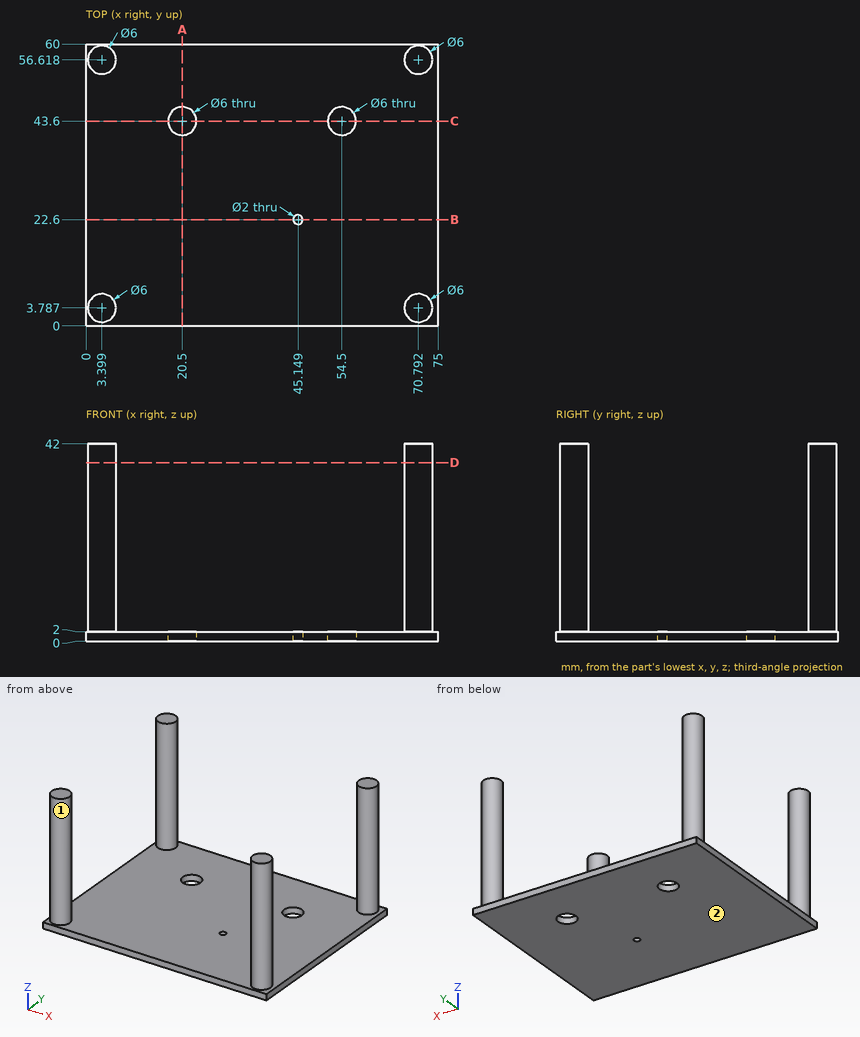
Verification items for this drawing (mm, ordinates from the low corner). Give positions to 0.01 mm unless a question says otherwise; leave off trailing zeros. Write each loop counter-clockwise with the first axis right and the second up, starting at its lowest first coordinate (ties: lowest second). Pieces come first, ordered by that corner, then holes. Notation, with made-up numbers: (-15, 79.5) -> (27, 79.5) arc R23 ccw to (27, 90.5) -> close; hole circle Ø4 at (44.25, 53). An arc over 180 degrees is marked (long way). Write item = value, one per line.
Item 1: Sectioned sample at A-A on x = 20.5. Record the boundary of the cut face in (y, z).
Output:
outline = (0, 0) -> (40.6, 0) -> (40.6, 2) -> (0, 2) -> close; (46.6, 0) -> (60, 0) -> (60, 2) -> (46.6, 2) -> close
Item 2: Sectioned sample at C-C on y = 43.6. Record the boundary of the cut face in (x, z).
Output:
outline = (0, 0) -> (17.5, 0) -> (17.5, 2) -> (0, 2) -> close; (23.5, 0) -> (51.5, 0) -> (51.5, 2) -> (23.5, 2) -> close; (57.5, 0) -> (75, 0) -> (75, 2) -> (57.5, 2) -> close
Item 3: Sectioned sample at D-D on z = 38. Record the boundary of the cut face in (x, y).
Output:
outline = circle Ø6 at (3.4, 3.79); circle Ø6 at (3.4, 56.62); circle Ø6 at (70.79, 3.79); circle Ø6 at (70.79, 56.62)
Item 4: Sectioned sample at B-B on y = 22.6. Record the boundary of the cut face in (x, z), and give its area (3 significant figures).
Output:
outline = (0, 0) -> (44.15, 0) -> (44.15, 2) -> (0, 2) -> close; (46.15, 0) -> (75, 0) -> (75, 2) -> (46.15, 2) -> close
area = 146 mm^2
Item 5: Scan lines: probe 1 along Y at (x, z) = (54.5, 1.15); probe 2 along Z at (x, y) = (71.5, 45); probe 3 along X at (y, z) = (5, 39) (1 decimal). Record each from-to range of solid material in increasing order. Write a range as from..to.
Output:
probe_1 = 0..40.6, 46.6..60
probe_2 = 0..2
probe_3 = 0.7..6.1, 68..73.5
Item 6: Release check for a two-part mould opening along X. For the marked faces 1 and 2 record: +X half, -X half, draft (parallel to the pull), parting line (faces both ways), or undercut.
Output:
face_1 = undercut
face_2 = draft
Item 7: Gauge pin test, flat ends, axial feed: pin 1 (18 mm diameter, centred on x = 34, y = 32, fed in from +Z); pin 2 (1 mm diameter, centred on y = 6.5, z = 29, fed in from -X). Record the tip position at first contact, or that the pin passes through.
Output:
pin_1 = 2
pin_2 = 1.37
